Work out the finished part from the listing and answer in its coordinate system (mm). Face numbers are marked on the shaded views. A direction names the side the tool comes from. Coordinates: 2 decimals unless noted, no trailing zeros. Order: outer loops, then holes, each group sorted by start corner. A loop starts at its lowest first (then second) coordinate and runs counter-clockwise, first axis right, second up. Notation, with made-up numbers: M 88,80 L 133,80 A12 ccw 133,98 Z; hole C 56,4.5 d4. An arc over 180 degrees is marked long. Use a Markdown table: item, result. Add a question column.
Solid Edge part; units mm, degrees
sketch "Sketch1" plane through (0, 0, 0) normal (1, 0, 0) x (0, 1, 0)
  line L0 (-50, 25) -> (-50, -25)
  line L1 (-50, -25) -> (50, -25)
  line L2 (50, -25) -> (50, 25)
  line L3 (50, 25) -> (-50, 25)
extrude "Protrusion1" add sketch "Sketch1" along normal blind 4
sketch "Sketch2" plane through (4, 0, 0) normal (1, 0, 0) x (0, 1, 0)
  line L0 (11, 19) -> (-11, 19)
  line L1 (-11, 19) -> (-11, 25)
  line L2 (-11, 25) -> (11, 25)
  line L3 (11, 25) -> (11, 19)
extrude "ExtrudedProtrusion_2" add sketch "Sketch2" along normal blind 103
sketch "Sketch3" plane through (55.5, 0, 19) normal (0, 0, -1) x (0, 1, 0)
  circle A0 centre (0, 39.5) radius 6.45
  circle A1 centre (0, 1.5) radius 3
extrude "ExtrudedCutout_1" cut sketch "Sketch3" against normal blind 28.1055
sketch "Sketch4" plane through (4, 0, 0) normal (1, 0, 0) x (0, 1, 0)
  circle A0 centre (-40, 0) radius 4
  circle A1 centre (40, 0) radius 4
extrude "Cutout1" cut sketch "Sketch4" against normal up to next
properties material "Stainless steel"
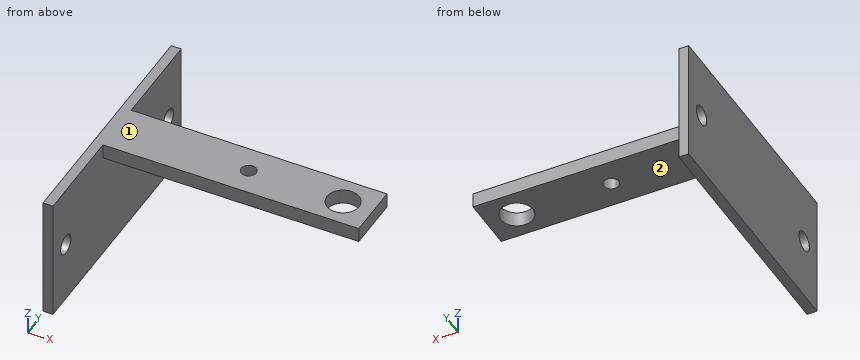
(1) Given P1, Ø10, axis at y = 3.5, z = -19, coming from the -X side; P2, Ø10, axis at y = 36.5, z = 14.5, coming from the +X side; P3, Ø6.5, axis at x = 65, z = 21, coming from the -Y side; P4, Ø24, axis at x = 74, y = 0, coming from the -Z side, each flat-ended and moving along its own axis, determine where each tip first touches the part or whether it passes through.
(2) A cutting plane is placed at B-B on x = 57. Write down the section's boundary in (y, z).
(3) Which of the six approach directions +Z, -Z, +X, -X, +Y, -Y give full straight-line access (tool end or side, diameter ignored) to the marked faces 1 and 2?
(4) Straight lines are drawn through the part: line 1 (X direction, y = 0, z = 21.1); line 2 (Z direction, x = 2.1, y = 40); line 3 (X direction, y = -31, z = -3.5). For each, find the intervals that lie inside material, in ascending order.
(5) A cutting plane is placed at C-C on y = -40. Write down the section's boundary in (x, z).
(6) A cutting plane is placed at D-D on y = 0. Write down the section's boundary in (x, z), plus the area to 3 significant figures.
(7) A cutting plane is placed at A-A on z = 0. Write down the section's boundary in (x, y).
From the geometry:
| question | item | result |
|---|---|---|
| 1 | P1 | stops at x = 0 |
| 1 | P2 | stops at x = 4 |
| 1 | P3 | stops at y = -11 |
| 1 | P4 | stops at z = 19 |
| 2 | outline | M -11,19 L -3,19 L -3,25 L -11,25 Z; M 3,19 L 11,19 L 11,25 L 3,25 Z |
| 3 | face 1 | +Z, +X, -X, +Y, -Y |
| 3 | face 2 | -Z, +X, +Y, -Y |
| 4 | line 1 | x = 0 to 54, 60 to 88.55, 101.45 to 107 |
| 4 | line 2 | z = -25 to -4, 4 to 25 |
| 4 | line 3 | x = 0 to 4 |
| 5 | outline | M 0,-25 L 4,-25 L 4,-4 L 0,-4 Z; M 0,4 L 4,4 L 4,25 L 0,25 Z |
| 6 | outline | M 0,-25 L 4,-25 L 4,19 L 54,19 L 54,25 L 0,25 Z; M 60,19 L 88.55,19 L 88.55,25 L 60,25 Z; M 101.45,19 L 107,19 L 107,25 L 101.45,25 Z |
| 6 | area | 705 mm2 |
| 7 | outline | M 0,-50 L 4,-50 L 4,-44 L 0,-44 Z; M 0,-36 L 4,-36 L 4,36 L 0,36 Z; M 0,44 L 4,44 L 4,50 L 0,50 Z |
